Model file for the job. Use its own axes, mm. A direction names the side the tool comes from. Round coordinates to 2 decimals unless told otherwise and drop trailing zeros. Loops run counter-clockwise (first coordinate to the right, second up) from the corner with the lowest first, then second, coordinate; pieces in that order, holes last. Notation, with made-up numbers: M -21.75,35 L 20.25,35 A28 cw 20.25,66 Z; hole C 57.25,-3.5 d8. An arc over 180 degrees is marked long. Use a Markdown table: item, result. Add a question column.
Q1. Probe line 1 (X direction, y = 9, z = 3.05) (3 decimals); line 2 (Y direction, x = 0, z = 1.05); line 3 (Y direction, x = 1, z = 2.05). List the from-to ranges inside material, lowest first. Write a range as from..to.
Q2. Cut at B-B (x = 10). Give the cut face in (y, z), plus the area to 3 significant figures.
Q3. Cut at A-A (z = 1.3). Give the cut face in (x, y).
Q4. Cut at D-D (x = 19.5). Give the cut face in (y, z).
Q5. Tool access for faces 4 (the face through (7, 0, 5)), 5 (the face through (25, 4.9, 2.5)): list every direction of +Z, -Z, +X, -X, +Y, -Y with a clear straight run to the whole face (end or side of a thin tool).
Q6. Mould opens along Y. For faces 1 (the face through (22.7, -10.8, 2.5)), 2 (the face through (7, 12.8, 2)), 3 (the face through (7, 0, 0)) say: +Y half, -Y half, draft (parallel to the pull), parting line (faces both ways), or undercut.
Q7. Cut at C-C (y = 8). Give the cut face in (x, z).
from build123d import *

# Parameters (mm, degrees)
ESQUISSE1_R             = 1.7
ESQUISSE1_R_2           = 2.6
BOSS_EXTRU_1_DEPTH      = 5
ENL_V_MAT_EXTRU_1_DEPTH = 3
ENL_V_MAT_EXTRU_1_TAPER = 5
CONG_1_R                = 4


with BuildPart() as part:
    # Esquisse1 → Boss.-Extru.1 (new body)
    with BuildSketch(Plane.XY):
        with BuildLine():
            Line((-12.8, -12.8), (12.8, -12.8))
            Line((12.8, -12.8), (26.514718626, -12.8))
            Line((26.514718626, -12.8), (26.514718626, -8.485281374))
            ThreePointArc((26.514718626, -8.485281374), (25.050252532, -4.949747468), (21.514718626, -3.485281374))
            ThreePointArc((21.514718626, -3.485281374), (18.029437252, 0), (21.514718626, 3.485281374))
            ThreePointArc((21.514718626, 3.485281374), (25.050252532, 4.949747468), (26.514718626, 8.485281374))
            Line((26.514718626, 8.485281374), (26.514718626, 12.8))
            Line((26.514718626, 12.8), (12.8, 12.8))
            Line((12.8, 12.8), (-12.8, 12.8))
            Line((-12.8, 12.8), (-12.8, -12.8))
        make_face()
        Circle(ESQUISSE1_R, mode=Mode.SUBTRACT)
        with Locations((-8.485281374, 8.485281374)):
            Circle(ESQUISSE1_R_2, mode=Mode.SUBTRACT)
        with Locations((8.485281374, 8.485281374)):
            Circle(ESQUISSE1_R_2, mode=Mode.SUBTRACT)
        with Locations((8.485281374, -8.485281374)):
            Circle(ESQUISSE1_R_2, mode=Mode.SUBTRACT)
        with Locations((-8.485281374, -8.485281374)):
            Circle(ESQUISSE1_R_2, mode=Mode.SUBTRACT)
        with Locations((21.514718626, -8.485281374)):
            Circle(ESQUISSE1_R_2, mode=Mode.SUBTRACT)
        with Locations((21.514718626, 8.485281374)):
            Circle(ESQUISSE1_R_2, mode=Mode.SUBTRACT)
    extrude(amount=BOSS_EXTRU_1_DEPTH)

    # Esquisse2 → Enlèv. mat.-Extru.1 (cut)
    with BuildSketch(Plane.XY.offset(5)):
        Polygon((3.233161507, 0), (1.616580754, 2.8), (-1.616580754, 2.8), (-3.233161507, 0), (-1.616580754, -2.8), (1.616580754, -2.8), align=None)
    extrude(amount=-ENL_V_MAT_EXTRU_1_DEPTH, taper=ENL_V_MAT_EXTRU_1_TAPER, mode=Mode.SUBTRACT)

    # Congé1
    cong_1_edges = [part.edges().sort_by_distance(p)[0] for p in [
        (26.514718626, 12.8, 2.5),
        (26.514718626, -12.8, 2.5),
        (-12.8, -12.8, 2.5),
        (-12.8, 12.8, 2.5),
    ]]
    fillet(cong_1_edges, radius=CONG_1_R)


solid = part.part
Checked values:
| question | item | result |
|---|---|---|
| 1 | line 1 | x = -12.795..-11.034, -5.937..5.937, 11.034..18.966, 24.063..26.51 |
| 1 | line 2 | y = -12.8..-1.7, 1.7..12.8 |
| 1 | line 3 | y = -12.8..-2.54, 2.54..12.8 |
| 2 | outline | M -12.8,0 L -10.6,0 L -10.6,5 L -12.8,5 Z; M -6.37,0 L 6.37,0 L 6.37,5 L -6.37,5 Z; M 10.6,0 L 12.8,0 L 12.8,5 L 10.6,5 Z |
| 2 | area | 85.7 mm^2 |
| 3 | outline | M -12.8,-8.8 A4 ccw -8.8,-12.8 L 22.51,-12.8 A4 ccw 26.51,-8.8 L 26.51,-8.49 A5 ccw 21.51,-3.49 A3.49 cw 21.51,3.49 A5 ccw 26.51,8.49 L 26.51,8.8 A4 ccw 22.51,12.8 L -8.8,12.8 A4 ccw -12.8,8.8 Z; hole C -8.49,-8.49 d5.2; hole C -8.49,8.49 d5.2; hole C 0,0 d3.4; hole C 8.49,-8.49 d5.2; hole C 8.49,8.49 d5.2; hole C 21.51,-8.49 d5.2; hole C 21.51,8.49 d5.2 |
| 4 | outline | M -12.8,0 L -10.13,0 L -10.13,5 L -12.8,5 Z; M -6.84,0 L -2.84,0 L -2.84,5 L -6.84,5 Z; M 2.84,0 L 6.84,0 L 6.84,5 L 2.84,5 Z; M 10.13,0 L 12.8,0 L 12.8,5 L 10.13,5 Z |
| 5 | face 4 | +Z, +X, -X, +Y, -Y |
| 5 | face 5 | +Z, -Z, +X |
| 6 | face 1 | undercut |
| 6 | face 2 | +Y half |
| 6 | face 3 | draft |
| 7 | outline | M -12.8,0 L -11.04,0 L -11.04,5 L -12.8,5 Z; M -5.93,0 L 5.93,0 L 5.93,5 L -5.93,5 Z; M 11.04,0 L 18.96,0 L 18.96,5 L 11.04,5 Z; M 24.07,0 L 26.49,0 L 26.49,5 L 24.07,5 Z |
